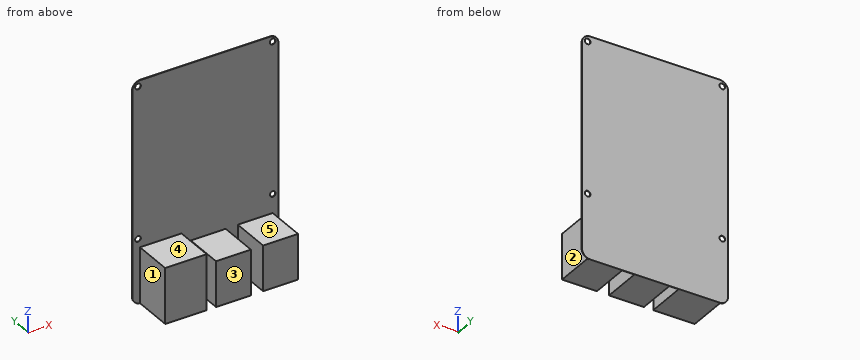
Autodesk Inventor part; units mm, degrees
ref_plane "YZ Plane" through (0, 0, 0) normal (1, 0, 0) x (0, 1, 0)
ref_plane "XZ Plane" through (0, 0, 0) normal (0, 1, 0) x (-1, 0, 0)
ref_plane "XY Plane" through (0, 0, 0) normal (0, 0, 1) x (1, 0, 0)
sketch "Sketch1" plane through (0, 0, 0) normal (0, 1, 0) x (-1, 0, 0)
  line L0 (28.4786, 33.7956) -> (-27.6046, 33.7956)
  line L1 (-27.6046, 33.7956) -> (-27.6046, -50.9896)
  line L2 (-27.6046, -50.9896) -> (28.4786, -50.9896)
  line L3 (28.4786, -50.9896) -> (28.4786, 33.7956)
  point P0 (0, 0)
  dimension "d0" = 56.0832
  dimension "d1" = 84.7852
extrude "Extrusion1" add sketch "Sketch1" along normal blind 0.1956
fillet "Fillet1" radius 3.175 4 edges at (27.6046, 0.0978, -50.9896) (-28.4786, 0.0978, -50.9896) (-28.4786, 0.0978, 33.7956) (27.6046, 0.0978, 33.7956)
sketch "Sketch2" plane through (0, 0, 0) normal (0, -1, 0) x (1, 0, 0)
  line L0 (-28.4786, -47.8146) -> (-28.4786, 30.6206) construction
  line L1 (-28.4786, 31.6112) -> (-26.2942, 31.6112) construction
  line L2 (-26.2942, 31.6112) -> (-26.2942, 33.7956) construction
  line L3 (-25.3036, 33.7956) -> (24.4296, 33.7956) construction
  circle A0 centre (-26.2942, 31.6112) radius 1.0922
  line L4 (27.6046, 30.6206) -> (27.6046, -47.8146) construction
  line L5 (27.6046, 31.6112) -> (25.4202, 31.6112) construction
  line L6 (25.4202, 31.6112) -> (25.4202, 33.7956) construction
  circle A1 centre (25.4202, 31.6112) radius 1.0922
  circle A2 centre (-26.2942, -26.3261) radius 1.0921
  circle A3 centre (25.4202, -26.3261) radius 1.0921
  point P0 (0, 0)
  dimension "d5" = 2.1844
  dimension "d6" = 2.1844
  dimension "d7" = 2.1844
  dimension "d8" = 2.1844
  dimension "d9" = 55.753
  dimension "d10" = 55.753
extrude "Extrusion2" cut sketch "Sketch2" against normal blind 0.1956
sketch "Sketch3" plane through (0, 0, 0) normal (0, -1, 0) x (1, 0, 0)
  line L0 (25.4202, -33.5906) -> (12.0344, -33.5906)
  line L1 (12.0344, -33.5906) -> (12.0344, -50.9896)
  line L2 (12.0344, -50.9896) -> (25.4202, -50.9896)
  line L3 (25.4202, -50.9896) -> (25.4202, -33.5906)
  line L4 (7.3354, -33.5906) -> (-6.0504, -33.5906)
  line L5 (-6.0504, -33.5906) -> (-6.0504, -50.9896)
  line L6 (-6.0504, -50.9896) -> (7.3354, -50.9896)
  line L7 (7.3354, -50.9896) -> (7.3354, -33.5906)
  line L8 (-25.5576, -29.7298) -> (-9.6318, -29.7298)
  line L9 (-9.6318, -29.7298) -> (-9.6318, -50.9896)
  line L10 (-9.6318, -50.9896) -> (-25.5576, -50.9896)
  line L11 (-25.5576, -50.9896) -> (-25.5576, -29.7298)
  line L12 (24.4296, -50.9896) -> (-25.3036, -50.9896)
  line L13 (27.6046, 30.6206) -> (27.6046, -47.8146)
  point P0 (0, 0)
  dimension "d13" = 13.3858
  dimension "d14" = 13.3858
  dimension "d16" = 17.399
  dimension "d18" = 21.2598
  dimension "d19" = 15.9258
  dimension "d20" = 0
  dimension "d21" = 0
  dimension "d22" = 4.699
  dimension "d23" = 3.5814
  dimension "d24" = 2.1844
extrude "Extrusion3" add sketch "Sketch3" along normal blind 15.24
equation "\"d6\" = d5"
equation "\"d7\" = d6"
equation "\"d8\" = d5"
equation "\"d10\" = d9"
equation "\"d14\" = d13"
properties part number "RPI"
Design review of the part built by this model. Coordinates are the model's own, in mm. Face numbers are marked on the shaded views. A direction names the side the tool comes from. Coordinates: 2 decimals unless noted, no trailing zeros. Loops run counter-clockwise (first coordinate to the right, second up) from the corner with the lowest first, then second, coordinate; pieces in that order, holes last. Notation, with made-up numbers: (88, -4) - (129, -4) arc R27 cw to (129, 19) - close; hole circle Ø6 at (56, 44.5). An arc over 180 degrees is marked (long way). Use CSV: the item, a comma, the result in double quotes. Start each with the question number.
1) Consider section C-C on x = -14. Write out the cut boundary in (y, z), then the cut area to 3 significant figures.
2) Consider section A-A on y = -13.5. Write out the cut boundary in (x, z).
3) Wall thickness on L1, parallel to X at y = -12.75, z = -40.5; L2, parallel to Z at x = 18, y = -2.5; L3, parallel to Z at x = -19, y = -11.25: over which ranges is each line inside the solid? List them lowest first. Write a range as from..to.
4) Consider section D-D on x = 9.5. Write out the cut boundary in (y, z).
5) Tool access review of the marked faces 1, 2, 3, 4 and 5: name each direction out of +Z, -Z, +X, -X, +Y, -Y from which nothing blocks a thin tool from reaching the whole face with its end or side.
6) Consider section B-B on z = -41. Write out the cut boundary in (x, y), then the cut area to 3 significant figures.
7) For pin 1 Ø8 at (x, y) = (-6, -10) entering from +Z; pin 2 Ø3 at (x, z) = (25.42, 31.61) entering from -Y; pin 3 Ø8 at (y, z) = (-2, 2.5) entering from +X; pin 4 Ø7.5 at (y, z) = (-5, -38) entering from +X, all flat-tipped, find the tip position at first contact; note any pin that passes through.
Geometry says:
1,outline,"(-15.24, -50.99) - (0.2, -50.99) - (0.2, 33.8) - (0, 33.8) - (0, -29.73) - (-15.24, -29.73) - close"
1,area,"341 mm^2"
2,outline,"(-25.56, -50.99) - (-9.63, -50.99) - (-9.63, -29.73) - (-25.56, -29.73) - close; (-6.05, -50.99) - (7.34, -50.99) - (7.34, -33.59) - (-6.05, -33.59) - close; (12.03, -50.99) - (25.42, -50.99) - (25.42, -33.59) - (12.03, -33.59) - close"
3,L1,"-25.56..-9.63, -6.05..7.34, 12.03..25.42"
3,L2,"-50.99..-33.59"
3,L3,"-50.99..-29.73"
4,outline,"(0, -50.99) - (0.2, -50.99) - (0.2, 33.8) - (0, 33.8) - close"
5,face 1,"+Z, -Z, -X, -Y"
5,face 2,"+Z, -Z, +X, -Y"
5,face 3,"+Z, -Z, +X, -X, -Y"
5,face 4,"+Z, +X, -X, -Y"
5,face 5,"+Z, +X, -Y"
6,outline,"(-28.48, 0) - (-25.56, 0) - (-25.56, -15.24) - (-9.63, -15.24) - (-9.63, 0) - (-6.05, 0) - (-6.05, -15.24) - (7.34, -15.24) - (7.34, 0) - (12.03, 0) - (12.03, -15.24) - (25.42, -15.24) - (25.42, 0) - (27.6, 0) - (27.6, 0.2) - (-28.48, 0.2) - close"
6,area,"662 mm^2"
7,pin 1,"z = -29.73"
7,pin 2,"y = 0"
7,pin 3,"x = 27.6"
7,pin 4,"x = 25.42"
